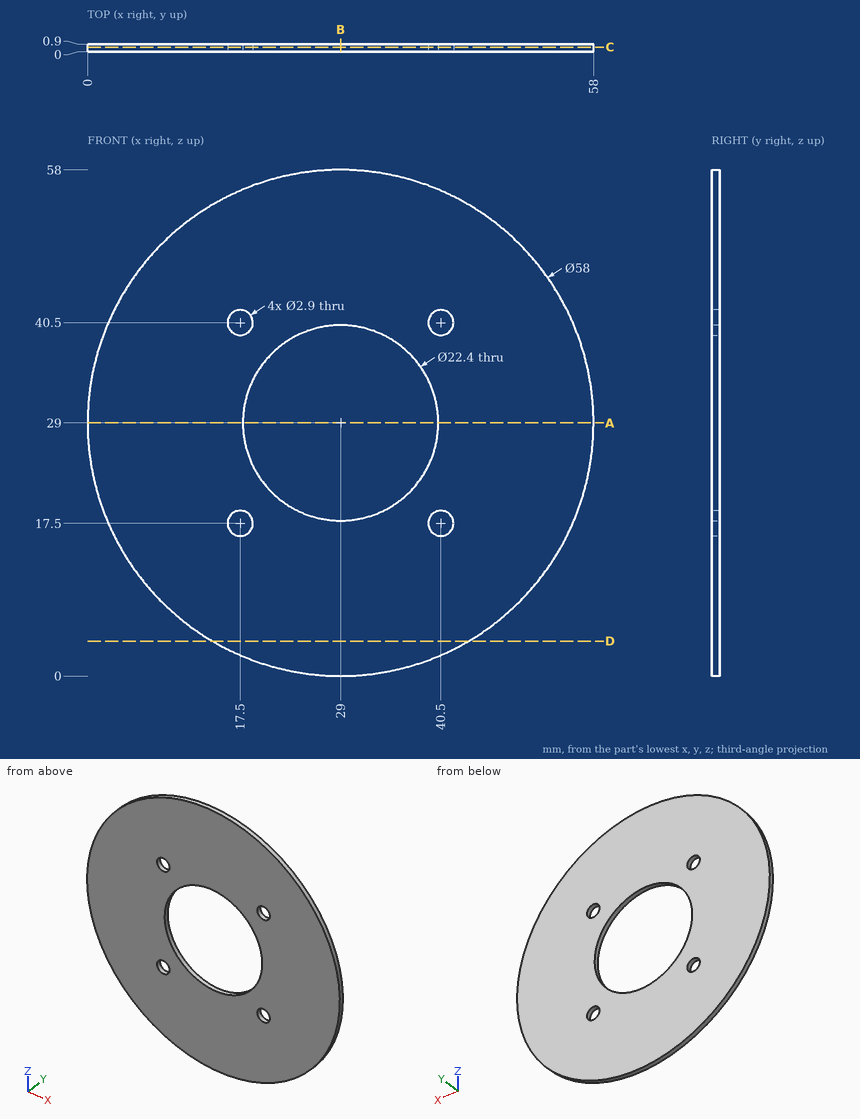
Can you work these out from the drawing? Everything is in mm from the part's minimum corner. Coordinates: 2 decimals unless noted, no trailing zeros. Write each loop counter-clockwise with the first axis right and the second up, starting at its lowest first coordinate (ties: lowest second). Pieces come first, ordered by that corner, then holes. Notation, with made-up numbers: (-36.75, -22) -> (17.25, -22) arc R15 cw to (17.25, -17) -> close; hole circle Ø10 at (38.5, 84). An arc over 180 degrees is marked (long way). Write item = value, one per line.
(1) For pin 1 (1.7 mm diameter, centred on x = 17.5, z = 40.5, fed in from +Y), with a flat end and sliding along its axis, tell me the tip position at first contact or that it passes through.
Verdict:
pin_1 = through
(2) Imagine slicing it at C-C (y = 0.55). Please give me the cut outline in (x, z), and give its area (3 significant figures).
Verdict:
outline = circle Ø58 at (29, 29); hole circle Ø2.9 at (17.5, 17.5); hole circle Ø2.9 at (17.5, 40.5); hole circle Ø22.4 at (29, 29); hole circle Ø2.9 at (40.5, 17.5); hole circle Ø2.9 at (40.5, 40.5)
area = 2,220 mm^2
(3) Imagine slicing it at A-A (z = 29). Please give me the cut outline in (x, y), and give its area (3 significant figures).
Verdict:
outline = (0, 0) -> (17.8, 0) -> (17.8, 0.9) -> (0, 0.9) -> close; (40.2, 0) -> (58, 0) -> (58, 0.9) -> (40.2, 0.9) -> close
area = 32.0 mm^2
(4) Imagine slicing it at D-D (z = 4). Please give me the cut outline in (x, y), and give its area (3 significant figures).
Verdict:
outline = (14.3, 0) -> (43.7, 0) -> (43.7, 0.9) -> (14.3, 0.9) -> close
area = 26.5 mm^2
(5) Imagine slicing it at B-B (x = 29). Please give me the cut outline in (y, z), and give its area (3 significant figures).
Verdict:
outline = (0, 0) -> (0.9, 0) -> (0.9, 17.8) -> (0, 17.8) -> close; (0, 40.2) -> (0.9, 40.2) -> (0.9, 58) -> (0, 58) -> close
area = 32.0 mm^2
(6) If I drill on probe 1 along X at (y, z) = (0.45, 17.5); probe 2 along X at (y, z) = (0.25, 41); probe 3 along Z at (x, y) = (41.5, 0.2), over which ranges is the centre line in solid material (lowest first)?
Verdict:
probe_1 = 2.38 to 16.05, 18.95 to 39.05, 41.95 to 55.62
probe_2 = 2.6 to 16.14, 18.86 to 39.14, 41.86 to 55.4
probe_3 = 2.83 to 16.45, 18.55 to 39.45, 41.55 to 55.17
